from build123d import *

# Parameters (mm, degrees)
BOSS_EXTRUDE1_DEPTH = 150
SHELL2_T            = -4
BOSS_EXTRUDE2_DEPTH = 150
FILLET1_R           = 2
SKETCH4_R           = 2.1
CUT_EXTRUDE1_DEPTH  = 150
SKETCH5_W           = 166
SKETCH5_H           = 2.845299462
BOSS_EXTRUDE3_DEPTH = 10
BOSS_EXTRUDE6_DEPTH = 150
FILLET2_R           = 2
SKETCH7_R           = 2.1
CUT_EXTRUDE3_DEPTH  = 150


with BuildPart() as part:
    # Sketch1 → Boss-Extrude1 (new body)
    with BuildSketch(Plane(origin=(0, 0, 0), x_dir=(1, 0, 0), z_dir=(0, 1, 0))):
        with BuildLine():
            Line((95, 0), (95, -69.582228732))
            ThreePointArc((95, -69.582228732), (90.839780928, -81.792934696), (80.089865986, -88.923719477))
            Line((80.089865986, -88.923719477), (5.089865986, -108.660561583))
            ThreePointArc((5.089865986, -108.660561583), (0, -109.319070837), (-5.089865986, -108.660561583))
            Line((-5.089865986, -108.660561583), (-80.089865986, -88.923719477))
            ThreePointArc((-80.089865986, -88.923719477), (-90.839780928, -81.792934696), (-95, -69.582228732))
            Line((-95, -69.582228732), (-95, 0))
            Line((-95, 0), (95, 0))
        make_face()
    extrude(amount=BOSS_EXTRUDE1_DEPTH)

    # Shell2
    shell2_openings = [part.faces().sort_by_distance(p)[0] for p in [
        (0, 150, 48.84344893),
        (0, 75, 0),
        (0, 0, 48.84344893),
    ]]
    offset(amount=SHELL2_T, openings=shell2_openings, kind=Kind.INTERSECTION)

    # Sketch3 → Boss-Extrude2 (add)
    with BuildSketch(Plane(origin=(0, 0, 0), x_dir=(1, 0, 0), z_dir=(0, 1, 0))):
        Polygon((-91, -4), (-83, -4), (-83, -8), (-91, -12.618802154), align=None)
        Polygon((-91, -69.582228732), (-76, -69.582228732), (-76, -85.863814167), (-80.300337087, -88.867104329), (-90.839780928, -81.792934696), (-95, -69.582228732), align=None)
        Polygon((91, -69.582228732), (76, -69.582228732), (76, -85.863814167), (80.300337087, -88.867104329), (90.839780928, -81.792934696), (95, -69.582228732), align=None)
        Polygon((83, -8), (91, -12.618802154), (91, -4), (83, -4), align=None)
    extrude(amount=BOSS_EXTRUDE2_DEPTH)

    # Fillet1
    fillet1_edges = [part.edges().sort_by_distance(p)[0] for p in [
        (83, 75, 8),
        (76, 75, 69.582228732),
        (-76, 75, 69.582228732),
        (-83, 75, 8),
    ]]
    fillet(fillet1_edges, radius=FILLET1_R)

    # Sketch4 → Cut-Extrude1 (cut)
    with BuildSketch(Plane(origin=(0, 0, 0), x_dir=(1, 0, 0), z_dir=(0, 1, 0))):
        with Locations(Location((84.197294702, -76.966150565, 0), (0, 0, 270))):
            Circle(SKETCH4_R)
        with Locations(Location((-84.197294702, -76.966150565, 0), (0, 0, 270))):
            Circle(SKETCH4_R)
    extrude(amount=CUT_EXTRUDE1_DEPTH, mode=Mode.SUBTRACT)

    # Sketch5 → Boss-Extrude3 (add)
    with BuildSketch(Plane(origin=(0, 0, 0), x_dir=(1, 0, 0), z_dir=(0, 1, 0))):
        with Locations((0, -5.422649731)):
            Rectangle(SKETCH5_W, SKETCH5_H)
    extrude(amount=BOSS_EXTRUDE3_DEPTH)

    # Sketch6 → Boss-Extrude6 (add)
    with BuildSketch(Plane(origin=(0, 0, 0), x_dir=(1, 0, 0), z_dir=(0, 1, 0))):
        Polygon((10, -97.119070837), (17.273176686, -101.318241355), (0, -107.972122026), (-17.273176686, -101.318241355), (-10, -97.119070837), align=None)
    extrude(amount=BOSS_EXTRUDE6_DEPTH)

    # Fillet2
    fillet2_edges = [part.edges().sort_by_distance(p)[0] for p in [
        (10, 75, 97.119070837),
        (-10, 75, 97.119070837),
        (-17.273176686, 75, 101.318241355),
        (17.273176686, 75, 101.318241355),
    ]]
    fillet(fillet2_edges, radius=FILLET2_R)

    # Sketch7 → Cut-Extrude3 (cut)
    with BuildSketch(Plane(origin=(0, 0, 0), x_dir=(1, 0, 0), z_dir=(0, 1, 0))):
        with Locations(Location((0, -103.219070837, 0), (0, 0, 270))):
            Circle(SKETCH7_R)
    extrude(amount=CUT_EXTRUDE3_DEPTH, mode=Mode.SUBTRACT)


solid = part.part
Design review of the part built by this model. Coordinates are the model's own, in mm. A direction names the side the tool comes from. Coordinates: 2 decimals unless noted, no trailing zeros. Loops run counter-clockwise (first coordinate to the right, second up) from the corner with the lowest first, then second, coordinate; pieces in that order, holes last. Notation, with made-up numbers: (7, -24.75) -> (39, -24.75) arc R10 ccw to (39, -8.75) -> close; hole circle Ø1 at (81, 8.5). An arc over 180 degrees is marked (long way). Use a Markdown table: item, result. Add a question column.
Item 1: The part is to be moulded in two halves that separate along Z. For faces 1 (the cylindrical face through (86.28, 73.95, 76.69)), 2 (the flat face through (-87.5, 74, 10.6)), 3 (the cylindrical face through (-90.727, 73.95, 81.938)), 4 (the flat face through (-93, 74, 0)), say which applies: +Z half, -Z half, draft (parallel to the pull), parting line (faces both ways), or undercut.
Item 2: We need section C-C, the plane y = 95. Count the separate pieces of the cut face and the enclosed holes in it, and give its area (3 significant figures).
Item 3: We need section A-A, the plane z = 42. Write out the cut boundary in (x, y), and give its area (3 significant figures).
Item 4: We need section B-B, the plane x = -34. Write out the cut boundary in (y, z), and give its area (3 significant figures).
Item 5: Clearance check with flat-ended pins moving along their axes: P1, Ø2.5, axis at x = 25, z = 5, coming from the +Y side; P2, Ø8, axis at x = -24, y = 58, coming from the +Z side; P3, Ø11.5, axis at y = 47, z = 77.5, coming from the -X side; P4, Ø2.5, axis at x = 84.2, z = 76.97, coming from the +Y side (3 decimals). State where each tip first meets the part, or that it passes through.
Item 6: Machinability: for faces 5 (the flat face through (95, 74, 34)), 6 (the flat face through (85, 74, 69.582)), 7 (the flat face through (91, 74, 2)), which of the approach directions +Z, -Z, +X, -X, +Y, -Y give a long, thin tool a straight path to every point of the face, cutting with its end or side? Answer none if there is none.
Item 7: Wall thickness on L1, parallel to X at y = 86, z = 47; L2, parallel to X at y = 94.5, z = 75.5; L3, parallel to Z at x = 82.5, y = 91: over which ranges is each line inside the solid? List them lowest first. Write a range as from..to.
Numbers:
| question | item | result |
|---|---|---|
| 1 | face 1 | undercut |
| 1 | face 2 | undercut |
| 1 | face 3 | +Z half |
| 1 | face 4 | -Z half |
| 2 | separate pieces | 1 |
| 2 | enclosed holes | 3 |
| 2 | area | 2,020 mm^2 |
| 3 | outline | (-95, 0) -> (-91, 0) -> (-91, 150) -> (-95, 150) -> close; (91, 0) -> (95, 0) -> (95, 150) -> (91, 150) -> close |
| 3 | area | 1,200 mm^2 |
| 4 | outline | (0, 4) -> (10, 4) -> (10, 6.85) -> (0, 6.85) -> close; (0, 96.92) -> (150, 96.92) -> (150, 101.05) -> (0, 101.05) -> close |
| 4 | area | 649 mm^2 |
| 5 | P1 | stops at y = 10 |
| 5 | P2 | stops at z = 104.74 |
| 5 | P3 | stops at x = -94.88 |
| 5 | P4 | passes through |
| 6 | face 5 | +Z, -Z, +X, +Y, -Y |
| 6 | face 6 | +Y, -Y |
| 6 | face 7 | -Z, +Y, -Y |
| 7 | L1 | x = -95..-91, 91..95 |
| 7 | L2 | x = -94.1..-85.7, -82.69..-76, 76..82.69, 85.7..94.1 |
| 7 | L3 | z = 69.58..75.73, 78.2..88.12 |
